The model under review builds one solid part; all positions refer to its coordinate system, in mm. Face numbers are marked on the shaded views. A direction names the side the tool comes from. Coordinates: 2 decimals unless noted, no trailing zeros. Loops run counter-clockwise (first coordinate to the right, second up) from the corner with the lowest first, then second, coordinate; pieces in that order, holes last. Notation, with made-up numbers: M 23,32 L 32,32 A15 cw 32,42 Z; hole C 74.5,-33 d9. An arc over 180 degrees is marked long. Return JSON: item names as keys, results as strings.
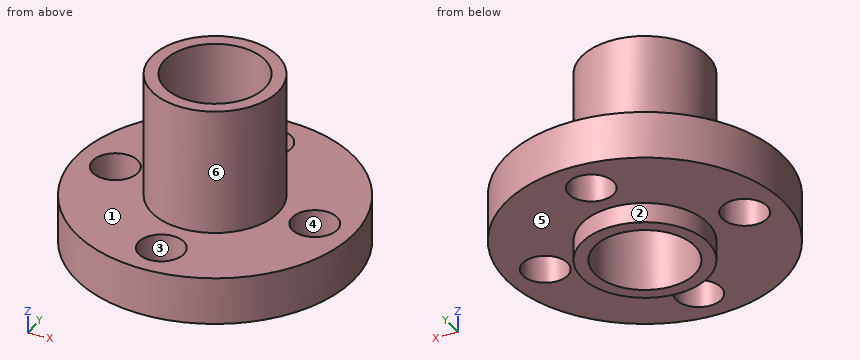
Autodesk Fusion 360 part; units mm, degrees
sketch "Sketch2" plane through (0, 0, 0) normal (0, 0, 1) x (1, 0, 0)
  circle A0 centre (0, 0) radius 5.05
  circle A1 centre (0, 0) radius 11.1
  line L0 (-35, 0) -> (41.5964, 0) construction
  line L1 (0, 35) -> (0, -35) construction
  circle A2 centre (0, 8) radius 1.8
  circle A3 centre (8, 0) radius 1.8
  circle A4 centre (0, -8) radius 1.8
  circle A5 centre (-8, 0) radius 1.8
  circle A6 centre (0, 0) radius 8 construction
  circle A7 centre (0, 0) radius 4
  dimension "d1" = 10.1
  dimension "d2" = 22.2
  dimension "d3" = 3.6
  dimension "d4" = 3.6
  dimension "d5" = 3.6
  dimension "d6" = 3.6
  dimension "d7" = 16
  dimension "d13" = 8
extrude "Extrude1" add sketch "Sketch2" along normal blind 15.5 contours A0 | A7
extrude "Extrude2" add sketch "Sketch2" along normal blind 3.8 from surface at 1.6 contours A1
extrude "Extrude3" cut sketch "Sketch2" along normal up to surface (15.5 mm away) contours A7
thread "Thread1"
1. Insertion check: pin 1 Ø4.5 at (x, y) = (0, 8) entering from -Z; pin 2 Ø2 at (x, y) = (-8, 0) entering from -Z; pin 3 Ø2 at (y, z) = (4.5, 12) entering from +X; pin 4 Ø3 at (y, z) = (3, 6) entering from +X. Each pin has a flat end and moves straight along its axis. Give the tip position at first contact, or say it passes through.
Check values:
{"pin 1": "z = 1.6", "pin 2": "through", "pin 3": "x = 3.64", "pin 4": "x = 10.98"}
2. Machinability: for the marked faces 1, 2 and 3, which of the approach directions +Z, -Z, +X, -X, +Y, -Y give a long, thin tool a straight path to every point of the face, cutting with its end or side? Answer none if there is none.
Check values:
{"face 1": "+Z", "face 2": "-Z", "face 3": "+Z, -Z"}
3. Add section C-C on z = 4.25. Give the boundary of the cut face in (x, y).
Check values:
{"outline": "C 0,0 d22.2; hole C -8,0 d3.6; hole C 0,0 d8; hole C 0,-8 d3.6; hole C 0,8 d3.6; hole C 8,0 d3.6"}
4. The part is to be moulded in two halves that separate along Y. For the marked faces 4, 5 and 6, say which applies: released by +Y, released by -Y, zero draft, split by the parting line, or undercut.
Check values:
{"face 4": "undercut", "face 5": "zero draft", "face 6": "split by the parting line"}
5. Add section A-A on y = 0. Give the boundary of the cut face in (x, z), plus the area to 3 significant figures.
Check values:
{"outline": "M -11.1,1.6 L -9.8,1.6 L -9.8,5.4 L -11.1,5.4 Z; M -6.2,1.6 L -5.05,1.6 L -5.05,0 L -4,0 L -4,15.5 L -5.05,15.5 L -5.05,5.4 L -6.2,5.4 Z; M 4,0 L 5.05,0 L 5.05,1.6 L 6.2,1.6 L 6.2,5.4 L 5.05,5.4 L 5.05,15.5 L 4,15.5 Z; M 9.8,1.6 L 11.1,1.6 L 11.1,5.4 L 9.8,5.4 Z", "area": "51.2 mm²"}
6. Add section B-B on x = -3.5. Give the boundary of the cut face in (y, z).
Check values:
{"outline": "M -10.53,1.6 L -3.64,1.6 L -3.64,0 L -1.94,0 L -1.94,15.5 L -3.64,15.5 L -3.64,5.4 L -10.53,5.4 Z; M 1.94,0 L 3.64,0 L 3.64,1.6 L 10.53,1.6 L 10.53,5.4 L 3.64,5.4 L 3.64,15.5 L 1.94,15.5 Z"}
7. To check wall thickness, follow line 1 (Y direction, x = 0, z = 4.1); line 2 (Y direction, x = 0, z = 6); line 3 (X direction, y = 7, z = 3.25). State the ranges of each line that lie inside material, in increasing order.
Check values:
{"line 1": "-11.1 to -9.8, -6.2 to -4, 4 to 6.2, 9.8 to 11.1", "line 2": "-5.05 to -4, 4 to 5.05", "line 3": "-8.61 to -1.5, 1.5 to 8.61"}
